Model file for the job. Use its own axes, mm. A direction names the side the tool comes from. Coordinates: 2 decimals unless noted, no trailing zeros. Loops run counter-clockwise (first coordinate to the right, second up) from the corner with the lowest first, then second, coordinate; pieces in that order, holes last. Notation, with made-up numbers: M -37,-18.5 L -23,-18.5 A12 ccw -23,0.5 Z; hole C -23.75,-28.75 d2. An arc over 180 degrees is marked long. Write item = value, one per line. Start each with the question number.
from build123d import *

# Parameters (mm, degrees)
F1_DEPTH = 25


with BuildPart() as f1:
    # F0 (on Top) → F1 (new body)
    with BuildSketch(Plane.XY):
        with BuildLine():
            ThreePointArc((306.79226, -127.929437), (311.81948, -115.792653), (323.956265, -110.765432))
            ThreePointArc((323.956265, -110.765432), (332.826212, -114.439485), (336.500265, -123.309432))
            ThreePointArc((336.500265, -123.309432), (330.500265, -129.309432), (324.500265, -123.309432))
            ThreePointArc((324.500265, -123.309432), (324.340931, -122.924766), (323.956265, -122.765432))
            ThreePointArc((323.956265, -122.765432), (320.304762, -124.277934), (318.79226, -127.929437))
            ThreePointArc((318.79226, -127.929437), (322.075007, -135.85469), (330.00026, -139.137437))
            ThreePointArc((330.00026, -139.137437), (345.477622, -132.719745), (351.872235, -117.232833))
            ThreePointArc((351.872235, -117.232833), (340.74764, -89.45185), (313.232341, -77.685459))
            ThreePointArc((313.232341, -77.685459), (265.575313, -97.462858), (245.84026, -145.137437))
            ThreePointArc((245.84026, -145.137437), (278.661963, -224.364314), (357.895707, -257.169435))
            ThreePointArc((357.895707, -257.169435), (491.315491, -202.202906), (547.341988, -69.224752))
            ThreePointArc((547.341988, -69.224752), (456.384064, 145.951907), (240.340265, 234.830562))
            ThreePointArc((240.340265, 234.830562), (-111.798912, 88.969739), (-257.659735, -263.169437))
            ThreePointArc((-257.659735, -263.169437), (-259.417094, -267.412078), (-263.659735, -269.169437))
            Line((-263.659735, -269.169437), (143.917844, -269.169437))
            Line((143.917844, -269.169437), (143.917844, -269.167725))
            ThreePointArc((143.917844, -269.167725), (138.370203, -265.466321), (139.669806, -258.925086))
            ThreePointArc((139.669806, -258.925086), (195.55159, -192.308055), (238.994524, -116.986649))
            ThreePointArc((238.994524, -116.986649), (240.92914, -112.33196), (243.155024, -107.809316))
            ThreePointArc((243.155024, -107.809316), (272.384887, -77.025709), (313.292265, -65.685432))
            ThreePointArc((313.292265, -65.685432), (349.277676, -81.011298), (363.872242, -117.299459))
            ThreePointArc((363.872242, -117.299459), (353.939349, -141.228584), (330.00026, -151.137437))
            ThreePointArc((330.00026, -151.137437), (313.589725, -144.339972), (306.79226, -127.929437))
        make_face()
    extrude(amount=-F1_DEPTH)


solid = f1.part
Item 1: Pin check, flat tips, straight feed: pin 1 Ø1.5 at (y, z) = (45, -6.5) entering from +X; pin 2 Ø6 at (x, z) = (399.5, -20) entering from -Y; pin 3 Ø2 at (y, z) = (2.5, -14.5) entering from -X. Stop position of each tip, or through.
Item 2: 3-axis set-ups, long thin cutter, end or side, ignore diameter. For faces 5 (the cylindrical face through (458.755, 143.578, -12.325)), 6 (the cylindrical face through (345.307, -132.889, -12.325)), 7 (the cylindrical face through (277.796, -223.488, -12.325)): which of +Z, -Z, +X, -X, +Y, -Y reach the whole face in a straight line?
Item 3: Pull direction X, two halves, no side cores. Call faces 1 (the flat face through (-63, -269.169, -12)), 2 (the cylindrical face through (489.84, -203.65, -12.32)), 3 (the cylindrical face through (194.85, -193.31, -12.32)), 4 (the cylindrical face through (-107.906, 92.82, -12.325)): +X half, -X half, draft (parallel to the pull), parting line (faces both ways), or undercut.
Item 4: Cut at D-D (y = 29). Give the cut face in (x, z).
Item 5: Probe L1, parallel to Y at x = 261, z = -8; L2, parallel to X at y = -83, z = -22.75; L3, parallel to X at y = -156, z = -15.25. List the from-to ranges inside material, lowest first.
Item 6: Cut at C-C (x = 122). Give the cut face in (y, z).
Item 7: Cut at A-A (y = -232.5). Give the cut face in (x, z).
Reported:
q1.pin_1 = 524.42
q1.pin_2 = -253.19
q1.pin_3 = -181.51
q2.face_5 = +Z, -Z, +X, +Y
q2.face_6 = +Z, -Z
q2.face_7 = +Z, -Z, -Y
q3.face_1 = draft
q3.face_2 = +X half
q3.face_3 = undercut
q3.face_4 = -X half
q4.outline = M -162.95,-25 L 530.2,-25 L 530.2,0 L -162.95,0 Z
q5.L1 = -201.41 to -102.53, -85.32 to 234.13
q5.L2 = -223.93 to 263.78, 287.05 to 332.48, 351.13 to 546.73
q5.L3 = -245.99 to 218.69, 246.37 to 525.51
q6.outline = M -269.17,-25 L 220.57,-25 L 220.57,0 L -269.17,0 Z
q7.outline = M -256.71,-25 L 164.25,-25 L 164.25,0 L -256.71,0 Z; M 287.74,-25 L 451.35,-25 L 451.35,0 L 287.74,0 Z
